```python
from build123d import *

# Parameters (mm, degrees)
EXTRUDE_1_DEPTH     = 10
EXTRUDE_2_DEPTH     = 5
CUT_EXTRUDE_2_DEPTH = 5


with BuildPart() as part:
    # 草图1 → 凸台-拉伸1 (new body)
    with BuildSketch(Plane.XY):
        Polygon((69.282032303, 0), (34.641016151, 60), (-34.641016151, 60), (-69.282032303, 0), (-34.641016151, -60), (34.641016151, -60), align=None)
    extrude(amount=EXTRUDE_1_DEPTH)

    # 草图2 → 凸台-拉伸2 (add)
    with BuildSketch(Plane(origin=(0, 0, 0), x_dir=(-1, 0, 0), z_dir=(0, 0, -1))):
        with BuildLine():
            Line((-16.163229875, 60), (16.163229875, 60))
            ThreePointArc((16.163229875, 60), (10.9905365, 62.959729742), (10.921101267, 68.918918919))
            ThreePointArc((10.921101267, 68.918918919), (0, 87.5), (-10.921101267, 68.918918919))
            ThreePointArc((-10.921101267, 68.918918919), (-10.9905365, 62.959729742), (-16.163229875, 60))
        make_face()
    extrude(amount=-EXTRUDE_2_DEPTH)

    # 草图3 → 切除-拉伸2 (cut)
    with BuildSketch(Plane(origin=(0, 0, 0), x_dir=(-1, 0, 0), z_dir=(0, 0, -1))):
        with BuildLine():
            ThreePointArc((-11.026755844, -51.096774194), (-11.109451344, -57.048003048), (-16.27759196, -60))
            Line((-16.27759196, -60), (0, -60))
            Line((0, -60), (16.27759196, -60))
            ThreePointArc((16.27759196, -60), (11.109451344, -57.048003048), (11.026755844, -51.096774194))
            ThreePointArc((11.026755844, -51.096774194), (0, -32.4), (-11.026755844, -51.096774194))
        make_face()
    extrude(amount=-CUT_EXTRUDE_2_DEPTH, mode=Mode.SUBTRACT)


solid = part.part
```
CAD build for the part. Positions are in the model's coordinates, mm. A direction names the side the tool comes from. Round coordinates to 2 decimals unless told otherwise and drop trailing zeros. Order: outer loops, then holes, each group sorted by start corner. A loop starts at its lowest first (then second) coordinate and runs counter-clockwise, first axis right, second up. Notation, with made-up numbers: (57.25, -9.5) -> (66.25, -9.5) arc R25 cw to (66.25, 18.5) -> close; hole circle Ø6 at (-28, -39.5). An arc over 180 degrees is marked (long way). Write item = value, one per line.
(1) Cut at A-A (x = 0). Write the cut outline in (y, z).
Answers follow:
outline = (-60, 5) -> (-32.4, 5) -> (-32.4, 0) -> (87.5, 0) -> (87.5, 5) -> (60, 5) -> (60, 10) -> (-60, 10) -> close
(2) Cut at B-B (z = 8). Write the cut outline in (x, y).
Answers follow:
outline = (-69.28, 0) -> (-34.64, -60) -> (34.64, -60) -> (69.28, 0) -> (34.64, 60) -> (-34.64, 60) -> close
(3) Cut at D-D (y = -45). Write the cut outline in (x, z).
Answers follow:
outline = (-43.3, 0) -> (-12.6, 0) -> (-12.6, 5) -> (12.6, 5) -> (12.6, 0) -> (43.3, 0) -> (43.3, 10) -> (-43.3, 10) -> close
(4) 3-axis set-ups, long thin cutter, end or side, ignore diameter. For faces 4 (the flat face through (0, -46, 5)), 5 (the flat face through (0, 74, 5)), 6 (the cylindrical face through (-11.04, 62.88, 2.46)): which of +Z, -Z, +X, -X, +Y, -Y reach the whole face in a straight line?
Answers follow:
face_4 = -Z
face_5 = +Z, +X, -X, +Y
face_6 = +Z, -Z, -X
(5) Flat gauge pins, fed straight in: P1, Ø5, axis at x = -9, z = 4, coming from the +Y side; P2, Ø22, axis at x = -4.5, y = 77.5, coming from the +Z side; P3, Ø6, axis at x = -48, z = 2.5, coming from the +Y side. Where does each tip first touch, or does it go through?
Answers follow:
P1 = 85.68
P2 = 5
P3 = 42.06
(6) Cut at C-C (y = 75). Write the cut outline in (x, z).
Answers follow:
outline = (-12.5, 0) -> (12.5, 0) -> (12.5, 5) -> (-12.5, 5) -> close
(7) Drill centre lines: L1, parallel to Y at x = 26, z = 1.75; L2, parallel to Y at x = 0, z = 3.55; L3, parallel to X at y = -45, z = 1.25. Where is each one in solid material? Low to high.
Answers follow:
L1 = -60 to 60
L2 = -32.4 to 87.5
L3 = -43.3 to -12.6, 12.6 to 43.3
(8) Pull direction Y, two halves, no side cores. Call faces 1 (the flat face through (51.72, -30.42, 4.93)), 2 (the flat face through (0, 60, 6)), 3 (the cylindrical face through (-11.154, -57.123, 2.465)): +Y half, -Y half, draft (parallel to the pull), parting line (faces both ways), or undercut.
Answers follow:
face_1 = -Y half
face_2 = +Y half
face_3 = undercut
